Drawing for the job (mm, zero at the part's lowest x, y, z). A direction names the side the tool comes from. Give positions to 0.01 mm unless a question says otherwise; leave off trailing zeros. Loops run counter-clockwise (first coordinate to the right, second up) from the corner with the lowest first, then second, coordinate; pieces in that order, holes last. Notation, with made-up numbers: (15, 22.25) - (60, 22.25) arc R18 ccw to (60, 42.25) - close; hole circle Ø6 at (13, 36.25). An arc over 180 degrees is marked (long way). Return JSON: item names as keys, results as strings. Group by question number.
1) Drop a flat-ended pin along its axis: pin 1 (2 mm diameter, centred on x = 19.5, z = 53, fed in from -Y). Give the stop position or say it passes through.
2) Slice it at C-C (z = 31). List the corners of the cut face in (x, y), and give its area (3 significant figures).
3) Drill centre lines: probe 1 along Y at (x, z) = (44, 110); probe 2 along X at (y, z) = (47.5, 153). Where is each one in solid material? Low to high. Write a range as from..to.
4) Mould opens along Y. For the marked faces 3, 4 and 5 say: released by +Y, released by -Y, zero draft, split by the parting line, or undercut.
5) Slice it at A-A (x = 40.5). List the corners of the cut face in (y, z), and give its area (3 significant figures).
6) 3-axis set-ups, long thin cutter, end or side, ignore diameter. For the marked faces 1 and 2: which of +Z, -Z, +X, -X, +Y, -Y reach the whole face in a straight line?
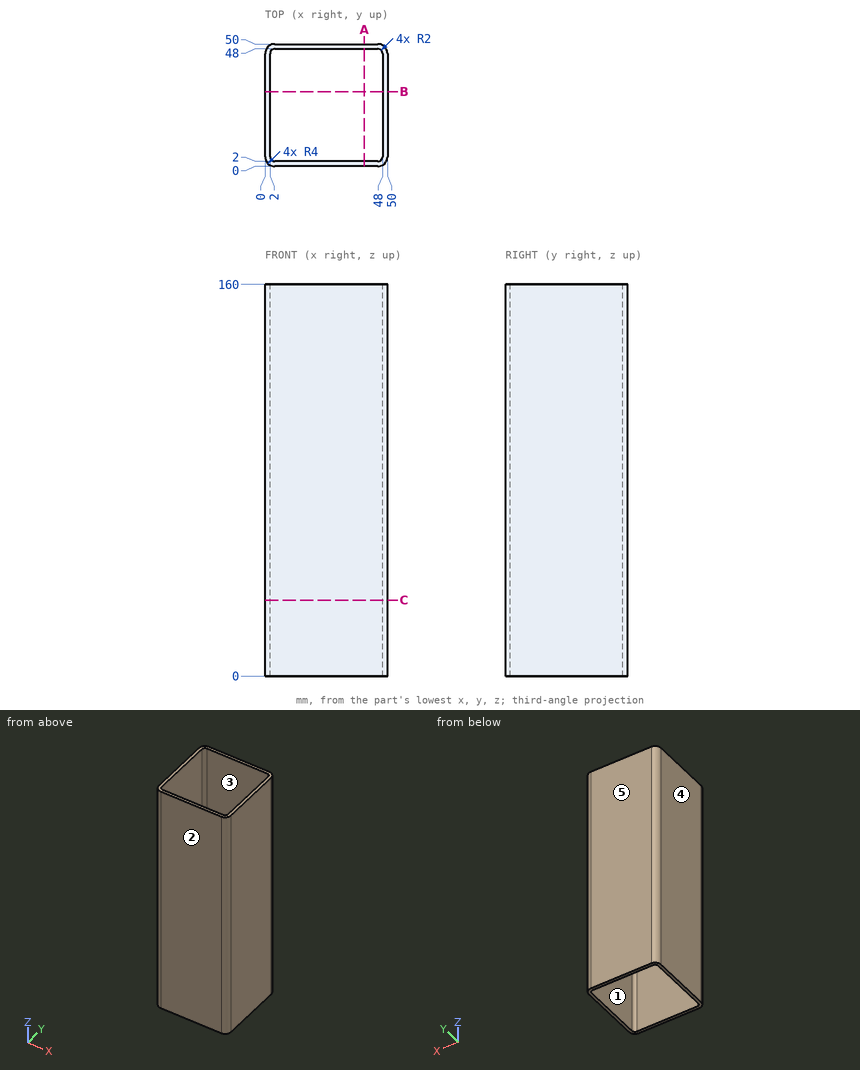
Results:
{
 "1": {"pin 1": "y = 0"},
 "2": {"outline": "(0, 4) arc R4 ccw to (4, 0) - (46, 0) arc R4 ccw to (50, 4) - (50, 46) arc R4 ccw to (46, 50) - (4, 50) arc R4 ccw to (0, 46) - close; hole (2, 4) arc R2 ccw to (4, 2) - (46, 2) arc R2 ccw to (48, 4) - (48, 46) arc R2 ccw to (46, 48) - (4, 48) arc R2 ccw to (2, 46) - close", "area": "374 mm2"},
 "3": {"probe 1": "0..2, 48..50", "probe 2": "0.29..2.68, 47.32..49.71"},
 "4": {"face 3": "undercut", "face 4": "zero draft", "face 5": "released by +Y"},
 "5": {"outline": "(0, 0) - (2, 0) - (2, 160) - (0, 160) - close; (48, 0) - (50, 0) - (50, 160) - (48, 160) - close", "area": "640 mm2"},
 "6": {"face 1": "+Z, -Z", "face 2": "+Z, -Z, +X, -X, -Y"}
}
